Here's how the part is built. I have some questions about the finished solid (model axes, mm). Face numbers are marked on the shaded views. A direction names the side the tool comes from. Round coordinates to 2 decimals unless told otherwise and drop trailing zeros. Write each loop counter-clockwise with the first axis right and the second up, starting at its lowest first coordinate (ties: lowest second). Pieces come first, ordered by that corner, then holes. Notation, with made-up numbers: (66.5, 18) - (105.5, 18) arc R27 ccw to (105.5, 37) - close; hole circle Ø4 at (-23, 41.25). An arc over 180 degrees is marked (long way). One line per item, written item: value. Start each with the question number.
Item 1: For P1, Ø2.5, axis at x = 0, y = 0, coming from the +Z side, with a flat end and sliding along its axis, tell me the tip position at first contact or that it passes through.
Item 2: Thinking about a two-plate mould opening in X: for the marked faces 1, 2 and 3, which applies, released by +X, released by -X, zero draft, split by the parting line, or undercut?
Item 3: If I drill on line 1 (Y direction, x = 0, z = 0.85); line 2 (Y direction, x = 0, z = 3.15); line 3 (Z direction, x = 2.25, y = -4.5), over which ranges is the centre line in solid material (lowest first)?
Item 4: Imagine slicing it at A-A, the plane x = 0. Please give me the cut outline in (y, z), then the cut area to 3 significant figures.
Item 5: For the marked faces 4 and 5, which set-ups out of +Z, -Z, +X, -X, +Y, -Y let a thin tool reach every point of the face, with its end or its side?
Item 6: Imagine slicing it at D-D, the plane y = 4.5. Please give me the cut outline in (x, z), then the cut area to 3 significant figures.
Item 7: Imagine slicing it at C-C, the plane z = 0.6. Please give me the cut outline in (x, y), then the cut area to 3 significant figures.
```python
from build123d import *

# Parameters (mm, degrees)
SKETCH1_W           = 12
SKETCH1_H           = 12
BOSS_EXTRUDE1_DEPTH = 2
SKETCH2_R           = 3
SKETCH2_R_2         = 2.5
BOSS_EXTRUDE2_DEPTH = 3
SKETCH5_R           = 1
CUT_EXTRUDE1_DEPTH  = 10


with BuildPart() as part:
    # Sketch1 → Boss-Extrude1 (new body)
    with BuildSketch(Plane.XY):
        Rectangle(SKETCH1_W, SKETCH1_H)
    extrude(amount=BOSS_EXTRUDE1_DEPTH)

    # Sketch2 → Boss-Extrude2 (add)
    with BuildSketch(Plane.XY.offset(2)):
        Circle(SKETCH2_R)
        Circle(SKETCH2_R_2, mode=Mode.SUBTRACT)
    extrude(amount=BOSS_EXTRUDE2_DEPTH)

    # Sketch5 → Cut-Extrude1 (cut, through all)
    with BuildSketch(Plane.XY.offset(2)):
        Circle(SKETCH5_R)
    extrude(amount=-CUT_EXTRUDE1_DEPTH, mode=Mode.SUBTRACT)


solid = part.part
```
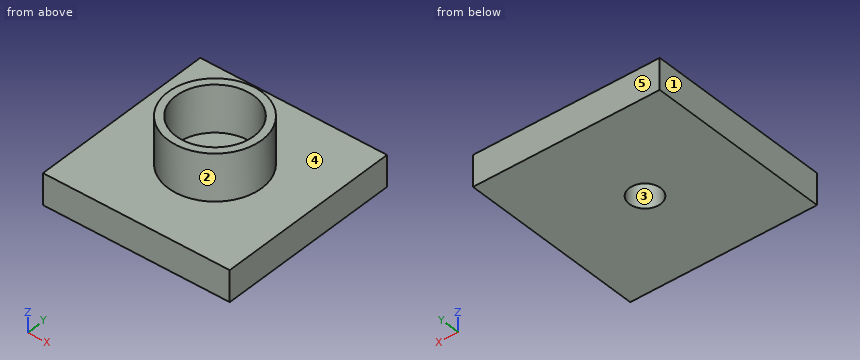
Values follow:
1. P1: stops at z = 2
2. face 1: released by -X
2. face 2: split by the parting line
2. face 3: undercut
3. line 1: y = -6 to -1, 1 to 6
3. line 2: y = -3 to -2.5, 2.5 to 3
3. line 3: z = 0 to 2
4. outline: (-6, 0) - (-1, 0) - (-1, 2) - (-2.5, 2) - (-2.5, 5) - (-3, 5) - (-3, 2) - (-6, 2) - close; (1, 0) - (6, 0) - (6, 2) - (3, 2) - (3, 5) - (2.5, 5) - (2.5, 2) - (1, 2) - close
4. area: 23.0 mm^2
5. face 4: +Z
5. face 5: +Z, -Z, +X, -X, +Y
6. outline: (-6, 0) - (6, 0) - (6, 2) - (-6, 2) - close
6. area: 24.0 mm^2
7. outline: (-6, -6) - (6, -6) - (6, 6) - (-6, 6) - close; hole circle Ø2 at (0, 0)
7. area: 141 mm^2
